Could you check a few things on this model? Use its own coordinates, in mm. Face numbers are marked on the shaded views. A direction names the side the tool comes from. Round coordinates to 2 decimals unless told otherwise and drop trailing zeros. Loops run counter-clockwise (first coordinate to the right, second up) from the corner with the lowest first, then second, coordinate; pieces in that order, holes last. Notation, with made-up numbers: (-25, -36.75) - (18, -36.75) arc R38 ccw to (18, 1.25) - close; hole circle Ø6 at (-30, 44.5). An arc over 180 degrees is marked (long way). Use one line per item in the form item = value.
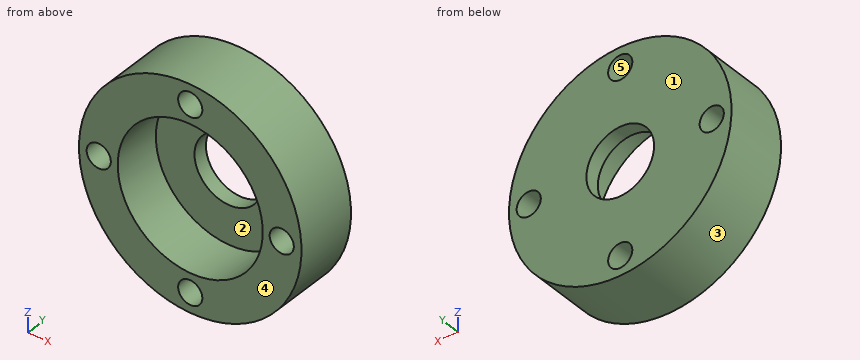
```python
from build123d import *

# Parameters (mm, degrees)
SKETCH_1_R          = 11.5
SKETCH_1_R_2        = 7.5
EXTRUDE_1_DEPTH     = 5
SKETCH_2_R          = 11.5
EXTRUDE_3_DEPTH     = 1.5
SKETCH_3_R          = 1.25
CUT_EXTRUDE_4_DEPTH = 18.514279888
SKETCH_4_R          = 3.5
CUT_EXTRUDE_5_DEPTH = 18.514279888


with BuildPart() as part:
    # Эскиз1 → Вытянуть1 (new body)
    with BuildSketch(Plane(origin=(0, 0, 0), x_dir=(1, 0, 0), z_dir=(0, 1, 0))):
        with Locations(Location((0, 0, 0), (0, 0, 270))):
            Circle(SKETCH_1_R)
        with Locations(Location((0, 0, 0), (0, 0, 270))):
            Circle(SKETCH_1_R_2, mode=Mode.SUBTRACT)
    extrude(amount=EXTRUDE_1_DEPTH)

    # Эскиз2 → Вытянуть3 (add)
    with BuildSketch(Plane(origin=(0, 5, 0), x_dir=(1, 0, 0), z_dir=(0, 1, 0))):
        with Locations(Location((0, 0, 0), (0, 0, 270))):
            Circle(SKETCH_2_R)
    extrude(amount=EXTRUDE_3_DEPTH)

    # Эскиз3 → Вытянуть4 (cut, through all)
    with BuildSketch(Plane(origin=(0, 6.5, 0), x_dir=(-1, 0, 0), z_dir=(0, 1, 0))):
        with Locations(Location((0, -9.45968553, 0), (0, 0, 90))):
            Circle(SKETCH_3_R)
        with Locations(Location((-9.45968553, 0, 0), (0, 0, 90))):
            Circle(SKETCH_3_R)
        with Locations(Location((0, 9.45968553, 0), (0, 0, 90))):
            Circle(SKETCH_3_R)
        with Locations(Location((9.45968553, 0, 0), (0, 0, 90))):
            Circle(SKETCH_3_R)
    extrude(amount=-CUT_EXTRUDE_4_DEPTH, mode=Mode.SUBTRACT)

    # Эскиз4 → Вытянуть5 (cut, through all)
    with BuildSketch(Plane(origin=(0, 6.5, 0), x_dir=(-1, 0, 0), z_dir=(0, 1, 0))):
        with Locations(Location((0, 0, 0), (0, 0, 90))):
            Circle(SKETCH_4_R)
    extrude(amount=-CUT_EXTRUDE_5_DEPTH, mode=Mode.SUBTRACT)


solid = part.part
```
1. We'd pull the mould along X, two halves only. Please class the marked faces 3, 4 and 5: +X half, -X half, draft (parallel to the pull), parting line (faces both ways), or undercut.
Solution:
face_3 = parting line
face_4 = draft
face_5 = undercut
2. If we section it at B-B, the plane x = 0: Write out the boundary of the cut face in (y, z), plus the area to 3 significant figures.
Solution:
outline = (0, -11.5) - (6.5, -11.5) - (6.5, -10.71) - (0, -10.71) - close; (0, -8.21) - (6.5, -8.21) - (6.5, -3.5) - (5, -3.5) - (5, -7.5) - (0, -7.5) - close; (0, 7.5) - (5, 7.5) - (5, 3.5) - (6.5, 3.5) - (6.5, 8.21) - (0, 8.21) - close; (0, 10.71) - (6.5, 10.71) - (6.5, 11.5) - (0, 11.5) - close
area = 31.5 mm^2
3. On a 3-axis mill with a long thin cutter (end or side, diameter ignored), from which of +Z, -Z, +X, -X, +Y, -Y can I reach the whole of each face in a straight line? I mean the marked faces 1 and 2. Say none if no direction works.
Solution:
face_1 = +Z, -Z, +X, -X, +Y
face_2 = -Y
4. Please list where these lines run through material, in increasing order: line 1 along X through (y, z) = (3.75, 0); line 2 along X through (y, z) = (5.25, -0.75); line 3 along Y through (x, z) = (-4.75, 5.75).
Solution:
line_1 = -11.5 to -10.71, -8.21 to -7.5, 7.5 to 8.21, 10.71 to 11.5
line_2 = -11.48 to -10.46, -8.46 to -3.42, 3.42 to 8.46, 10.46 to 11.48
line_3 = 5 to 6.5
5. If we section it at A-A, the plane z = 0: Write out the boundary of the cut face in (x, y).
Solution:
outline = (-11.5, 0) - (-10.71, 0) - (-10.71, 6.5) - (-11.5, 6.5) - close; (-8.21, 0) - (-7.5, 0) - (-7.5, 5) - (-3.5, 5) - (-3.5, 6.5) - (-8.21, 6.5) - close; (3.5, 5) - (7.5, 5) - (7.5, 0) - (8.21, 0) - (8.21, 6.5) - (3.5, 6.5) - close; (10.71, 0) - (11.5, 0) - (11.5, 6.5) - (10.71, 6.5) - close
6. If we section it at C-C, the plane y = 5.75: Write out the boundary of the cut face in (x, z), plus the area to 3 significant figures.
Solution:
outline = circle Ø23 at (0, 0); hole circle Ø2.5 at (-9.46, 0); hole circle Ø7 at (0, 0); hole circle Ø2.5 at (0, -9.46); hole circle Ø2.5 at (0, 9.46); hole circle Ø2.5 at (9.46, 0)
area = 357 mm^2
7. If we section it at D-D, the plane x = 9: Write out the boundary of the cut face in (y, z).
Solution:
outline = (0, -7.16) - (6.5, -7.16) - (6.5, -1.16) - (0, -1.16) - close; (0, 1.16) - (6.5, 1.16) - (6.5, 7.16) - (0, 7.16) - close
8. For P1, Ø2, axis at x = -6, y = 2.5, coming from the -Z side; P2, Ø1, axis at x = 2, y = 3, coming from the +Z side; P3, Ø1, axis at x = 8, y = 3, coming from the +Z side, each with a flat end and sliding along its axis, tell me the tip position at first contact or that it passes through.
Solution:
P1 = -10.36
P2 = 11.4
P3 = 8.72
